Could you check a few things on this model? Use its own coordinates, in mm. A direction names the side the tool comes from. Give positions to 0.01 mm unless a question says otherwise; leave off trailing zeros. Order: outer loops, then holes, each group sorted by start corner. A loop starts at its lowest first (then second) coordinate and runs counter-clockwise, first axis right, second up. Notation, with made-up numbers: M 30.5,53.5 L 86.5,53.5 A23 ccw 86.5,81.5 Z; hole C 37.5,4.5 d1. An arc over 180 degrees is marked long. Use a Markdown table: item, result. Add a question column.
Item 1: If I drill on L1, parallel to Z at x = -18, y = 10; L2, parallel to Z at x = -42.5, y = 27; L3, parallel to Z at x = -18, y = 48, over which ranges is the centre line in solid material (lowest first)? Write a range as from..to.
Item 2: Suppose I cut it at A-A on x = -32. Write out the boundary of the cut face in (y, z), plus the area to 3 significant figures.
Item 3: Suppose I cut it at C-C on z = 24. Write out the boundary of the cut face in (x, y), plus the area to 3 significant figures.
Item 4: I'm going to push flat-ended pins straight in: pin 1 Ø5 at (y, z) = (50, -74.65) entering from +X; pin 2 Ø2 at (x, y) = (-40.5, 13.5) entering from +Z; pin 3 Ø24 at (y, z) = (14, -39.51) entering from +X; pin 4 Ø4 at (x, y) = (-20, 16) entering from -Z. Where does each tip first touch, or does it pass through?
Item 5: Suppose I cut it at B-B on y = 14. Write out the boundary of the cut face in (x, z), plus the area to 3 significant figures.
Item 6: For faces 1 (the face through (-17.04, 29.58, -71.41)), 2 (the face through (-18.098, 11.339, 58.375)), 3 (the face through (-38, 30, 48.99)), which set-ups out of +Z, -Z, +X, -X, +Y, -Y let a thin tool reach every point of the face, with its end or its side?
Item 7: Suppose I cut it at D-D on y = 27. Write out the boundary of the cut face in (x, z), plus the area to 3 significant figures.
Item 8: If we mould it in two halves opening along Y, with no side actions, what happens to faces 4 (the face through (-38, 30, -67.01)), 5 (the face through (-55, 0, -9)), 6 (the face through (-54.62, 11.13, 28.42))? For each: released by +Y, released by -Y, zero draft, split by the parting line, or undercut.
from build123d import *

# Parameters (mm, degrees)
EXTRUDE_1_DEPTH     = 60
SKETCH_3_W          = 110
SKETCH_3_H          = 60
CUT_EXTRUDE_1_DEPTH = 37
SKETCH_4_R          = 7.5
SKETCH_4_R_2        = 8.25
CUT_EXTRUDE_2_DEPTH = 5
SKETCH_7_R          = 2.2
CUT_EXTRUDE_3_DEPTH = 20
SKETCH_7_2_R        = 2.2
CUT_EXTRUDE_4_DEPTH = 9


with BuildPart() as part:
    # Sketch 2 → Extrude 1 (new body)
    with BuildSketch(Plane(origin=(0, 0, 0), x_dir=(1, 0, 0), z_dir=(0, 1, 0))):
        with BuildLine():
            Line((-19.040504883, -60.990225421), (-16.009924796, -60.990225421))
            ThreePointArc((-16.009924796, -60.990225421), (-19.758334463, -26.07939754), (-21.009924796, 9.009774579))
            ThreePointArc((-21.009924796, 9.009774579), (-19.758334463, 44.098946698), (-16.009924796, 79.009774579))
            Line((-16.009924796, 79.009774579), (-19.040504883, 79.009774579))
            ThreePointArc((-19.040504883, 79.009774579), (-19.858720594, 73.014546807), (-20.603665866, 67.009774579))
            Line((-20.603665866, 67.009774579), (-55.603665866, 67.009774579))
            Line((-55.603665866, 67.009774579), (-55.603665866, -48.990225421))
            Line((-55.603665866, -48.990225421), (-20.603665866, -48.990225421))
            ThreePointArc((-20.603665866, -48.990225421), (-19.858720594, -54.99499765), (-19.040504883, -60.990225421))
        make_face()
    extrude(amount=EXTRUDE_1_DEPTH)

    # Sketch 3 → Cut-Extrude 1 (cut)
    with BuildSketch(Plane.ZY.offset(16.603665866)):
        with Locations((-9.009774579, 30)):
            Rectangle(SKETCH_3_W, SKETCH_3_H)
    extrude(amount=CUT_EXTRUDE_1_DEPTH, mode=Mode.SUBTRACT)

    # Sketch 4 → Cut-Extrude 2 (cut)
    with BuildSketch(Plane.ZY.offset(55.603665866)):
        with Locations((21.490225421, 14)):
            Circle(SKETCH_4_R)
        with Locations((-39.509774579, 14)):
            Circle(SKETCH_4_R)
        with Locations((3.990225421, 43)):
            Circle(SKETCH_4_R_2)
        with Locations((-22.009774579, 43)):
            Circle(SKETCH_4_R_2)
    extrude(amount=-CUT_EXTRUDE_2_DEPTH, mode=Mode.SUBTRACT)

    # Sketch 7 → Cut-Extrude 3 (cut)
    with BuildSketch(Plane.ZY.offset(16.603665866)):
        with Locations(Location((-74.648328965, 50, 0), (0, 0, 180))):  # turned: the seam where the file's is
            Circle(SKETCH_7_R)
        with Locations(Location((-74.648328965, 10, 0), (0, 0, 180))):  # turned: the seam where the file's is
            Circle(SKETCH_7_R)
        with Locations(Location((56.628779808, 50, 0), (0, 0, 180))):  # turned: the seam where the file's is
            Circle(SKETCH_7_R)
        with Locations(Location((56.628779808, 10, 0), (0, 0, 180))):  # turned: the seam where the file's is
            Circle(SKETCH_7_R)
    extrude(amount=CUT_EXTRUDE_3_DEPTH, mode=Mode.SUBTRACT)

    # Sketch 7_2 → Cut-Extrude 4 (cut)
    with BuildSketch(Plane.ZY.offset(16.603665866)):
        with Locations(Location((-74.648328965, 50, 0), (0, 0, 180))):  # turned: the seam where the file's is
            Circle(SKETCH_7_2_R)
        with Locations(Location((-74.648328965, 10, 0), (0, 0, 180))):  # turned: the seam where the file's is
            Circle(SKETCH_7_2_R)
        with Locations(Location((56.628779808, 50, 0), (0, 0, 180))):  # turned: the seam where the file's is
            Circle(SKETCH_7_2_R)
        with Locations(Location((56.628779808, 10, 0), (0, 0, 180))):  # turned: the seam where the file's is
            Circle(SKETCH_7_2_R)
    extrude(amount=-CUT_EXTRUDE_4_DEPTH, mode=Mode.SUBTRACT)


solid = part.part
Findings below:
| question | item | result |
|---|---|---|
| 1 | L1 | z = -79.01..-76.85, -72.45..-64.01, 45.99..54.43, 58.83..60.99 |
| 1 | L2 | z = -67.01..-64.01, 45.99..48.99 |
| 1 | L3 | z = -79.01..-75.56, -73.73..-64.01, 45.99..55.71, 57.55..60.99 |
| 2 | outline | M 0,-67.01 L 60,-67.01 L 60,-64.01 L 0,-64.01 Z; M 0,45.99 L 60,45.99 L 60,48.99 L 0,48.99 Z |
| 2 | area | 360 mm^2 |
| 3 | outline | M -55.6,0 L -53.6,0 L -53.6,6.93 L -55.6,6.93 Z; M -55.6,21.07 L -53.6,21.07 L -53.6,60 L -55.6,60 Z |
| 3 | area | 91.7 mm^2 |
| 4 | pin 1 | stops at x = -16.27 |
| 4 | pin 2 | stops at z = 48.99 |
| 4 | pin 3 | stops at x = -53.6 |
| 4 | pin 4 | stops at z = -79.01 |
| 5 | outline | M -55.6,-67.01 L -20.6,-67.01 A495.5 ccw -19.04,-79.01 L -16.01,-79.01 A492.5 cw -17.93,-64.01 L -53.6,-64.01 L -53.6,-47.01 L -55.6,-47.01 Z; M -55.6,-32.01 L -53.6,-32.01 L -53.6,13.99 L -55.6,13.99 Z; M -55.6,28.99 L -53.6,28.99 L -53.6,45.99 L -17.93,45.99 A492.5 cw -16.01,60.99 L -19.04,60.99 A495.5 ccw -20.6,48.99 L -55.6,48.99 Z |
| 5 | area | 460 mm^2 |
| 6 | face 1 | +X, +Y, -Y |
| 6 | face 2 | +X, -X |
| 6 | face 3 | +Z, -X, +Y, -Y |
| 7 | outline | M -55.6,-67.01 L -20.6,-67.01 A495.5 ccw -19.04,-79.01 L -16.01,-79.01 A492.5 cw -17.93,-64.01 L -53.6,-64.01 L -53.6,45.99 L -17.93,45.99 A492.5 cw -16.01,60.99 L -19.04,60.99 A495.5 ccw -20.6,48.99 L -55.6,48.99 Z |
| 7 | area | 520 mm^2 |
| 8 | face 4 | zero draft |
| 8 | face 5 | released by -Y |
| 8 | face 6 | undercut |
